For this review, use the dimensioned drawing (mm, ordinates from the lowest corner) and the shaded views. A direction names the side the tool comes from. Coordinates: 2 decimals unless noted, no trailing zeros. Order: outer loops, then holes, each group sorted by start corner. A loop starts at its lowest first (then second) coordinate and runs counter-clockwise, first axis right, second up. Notation, with made-up numbers: M 78,52 L 116,52 A27 ccw 116,74 Z; hole C -5.75,60 d7. An arc over 180 degrees is marked long. Answer as CSV lines item,"result". Start each with the question number.
Q1. Consider section A-A on z = 68.5. Write out the cut boundary in (x, y) (1 decimal).
Q2. The part is to be moulded in two halves that separate along X. For the marked faces 1, 2 and 3, say which applies: +X half, -X half, draft (parallel to the pull), parting line (faces both ways), or undercut.
Q3. Machinability: for the marked faces 4 and 5, which of the approach directions +Z, -Z, +X, -X, +Y, -Y give a long, thin tool a straight path to every point of the face, cutting with its end or side? Answer none if there is none.
Q4. Consider section B-B on x = 7.5. Write out the cut boundary in (y, z) (1 decimal).
Q5. Consider section C-C on y = 20.25. Write out the cut boundary in (x, z).
Q6. Wall thickness on L1, parallel to X at y = 9, z = 72; L2, parallel to Y at x = 9.5, z = 49.5 (1 decimal): over which ranges is each line inside the solid? List them lowest first. Write a range as [from, to].
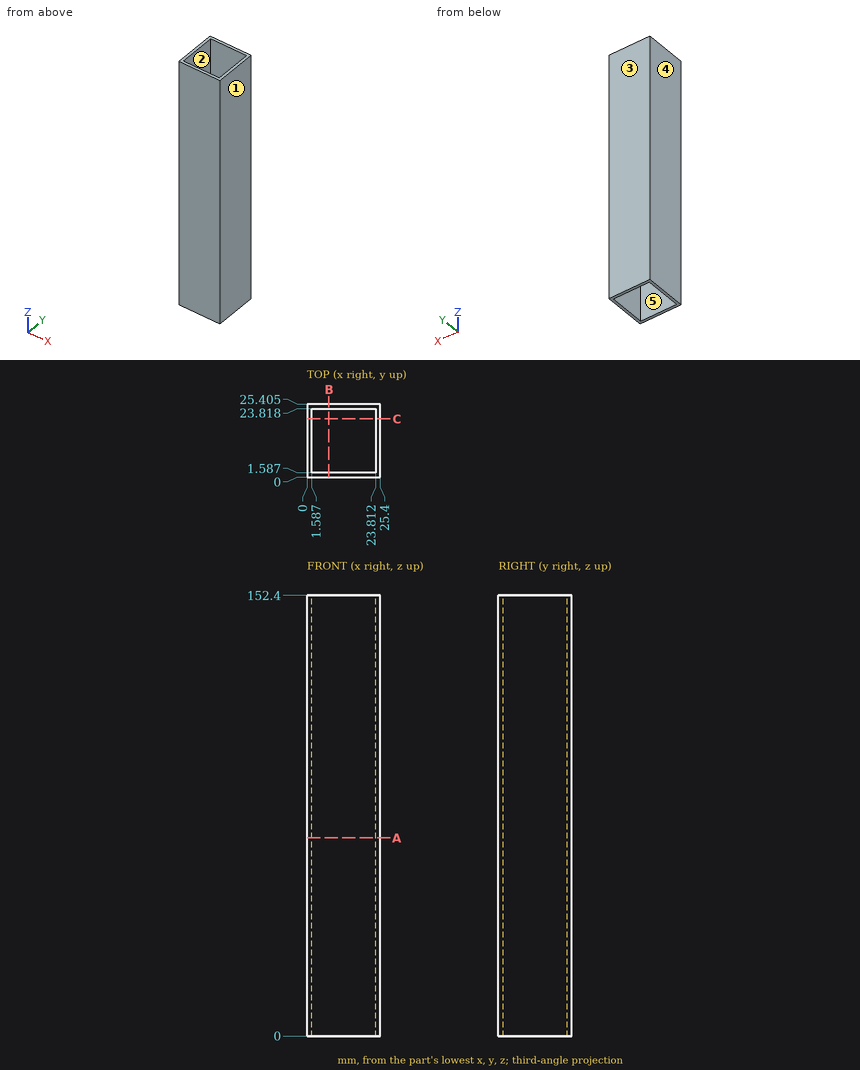
Evaluation:
1,outline,"M 0,0 L 25.4,0 L 25.4,25.4 L 0,25.4 Z; hole M 1.6,1.6 L 23.8,1.6 L 23.8,23.8 L 1.6,23.8 Z"
2,face 1,"+X half"
2,face 2,"undercut"
2,face 3,"draft"
3,face 4,"+Z, -Z, -X, +Y, -Y"
3,face 5,"+Z, -Z"
4,outline,"M 0,0 L 1.6,0 L 1.6,152.4 L 0,152.4 Z; M 23.8,0 L 25.4,0 L 25.4,152.4 L 23.8,152.4 Z"
5,outline,"M 0,0 L 1.59,0 L 1.59,152.4 L 0,152.4 Z; M 23.81,0 L 25.4,0 L 25.4,152.4 L 23.81,152.4 Z"
6,L1,"x = [0, 1.59], [23.81, 25.4]"
6,L2,"y = [0, 1.6], [23.8, 25.4]"
